Autodesk Inventor part; units mm, degrees
ref_plane "YZ Plane" through (0, 0, 0) normal (1, 0, 0) x (0, 1, 0)
ref_plane "XZ Plane" through (0, 0, 0) normal (0, 1, 0) x (-1, 0, 0)
ref_plane "XY Plane" through (0, 0, 0) normal (0, 0, 1) x (1, 0, 0)
sketch "Sketch1" plane through (0, 0, 0) normal (0, 0, 1) x (1, 0, 0)
  line L0 (0, 0) -> (30, 0)
  line L1 (0, 0) -> (0, 5)
  line L2 (0, 5) -> (30, 5)
  line L3 (30, 5) -> (30, 0)
  line L4 (30, 5) -> (30, 40)
  line L5 (30, 40) -> (33, 40)
  line L6 (33, 40) -> (33, 0)
  line L7 (33, 0) -> (30, 0)
  point P0 (23.0555, 5)
  dimension "d0" = 30
  dimension "d2" = 5
  dimension "d11" = 35
  dimension "d12" = 3
extrude "Extrusion1" add sketch "Sketch1" along normal blind 12
sketch "Sketch2" plane through (0, 0, 0) normal (0, -1, 0) x (1, 0, 0)
  circle A0 centre (25.8, 7) radius 2.125
  line L0 (33, 0) -> (33, 12)
  line L1 (0, 12) -> (33, 12)
  circle A1 centre (13.1, 7) radius 2.125
  point P0 (0, 0)
  point P1 (33, 6)
  dimension "d13" = 4.25
  dimension "d14" = 7.2
  dimension "d15" = 5
  dimension "d23" = 4.25
  dimension "d24" = 19.9
  dimension "d25" = 5
hole "Hole1" at (25.8, 0, 7) at (13.1, 0, 7) direction (0, 1, 0) diameter 5 end through all
properties part number "Support"
The model under review builds one solid part; all positions refer to its coordinate system, in mm. A direction names the side the tool comes from. Give positions to 0.01 mm unless a question says otherwise; leave off trailing zeros. Order: outer loops, then holes, each group sorted by start corner. A loop starts at its lowest first (then second) coordinate and runs counter-clockwise, first axis right, second up. Notation, with made-up numbers: (-39, 40) -> (-26, 40) arc R18 ccw to (-26, 56) -> close; hole circle Ø3 at (74, 24.25). An arc over 180 degrees is marked (long way). Write item = value, one per line. Start each with the question number.
(1) For L1, parallel to X at y = 2.85, z = 7; L2, parallel to Z at x = 13.1, y = 3.8; L3, parallel to X at y = 3.5, z = 5.25, list the stretches that pass through material, from the lowest coordinate up. Write a range as from..to.
(2) Take a section at D-D (y = 16). Write out the cut boundary in (x, z), plus the area to 3 significant figures.
(3) Take a section at B-B (z = 7). Write out the cut boundary in (x, y).
(4) Take a section at C-C (z = 1.25). Write out the cut boundary in (x, y).
(5) For pin 1 Ø3 at (x, z) = (13.1, 7) entering from -Y; pin 2 Ø6 at (y, z) = (31, 5.5) entering from -X; pin 3 Ø3.5 at (x, z) = (14, 8.5) entering from +Y, all flat-tipped, find the tip position at first contact; note any pin that passes through.
(6) Tool access review of faces 4 (the flat face through (30, 22, 6)), 5 (the flat face through (0, 2, 6)): name each direction out of +Z, -Z, +X, -X, +Y, -Y from which nothing blocks a thin tool from reaching the whole face with its end or side.
(7) Take a section at A-A (x = 25.8). Write out the cut boundary in (y, z).
(8) Draft analysis for pull direction Z (two halves, no side actions). For faces 1 (the cylindrical face through (12.349, 2.535, 4.615)), 2 (the flat face through (33, 20, 6)), 3 (the flat face through (23, 4, 0)), state which applies: +Z half, -Z half, draft (parallel to the pull), parting line (faces both ways), or undercut.
Returned:
q1.L1 = 0..10.6, 15.6..23.3, 28.3..33
q1.L2 = 0..4.5, 9.5..12
q1.L3 = 0..11.31, 14.89..24.01, 27.59..33
q2.outline = (30, 0) -> (33, 0) -> (33, 12) -> (30, 12) -> close
q2.area = 36.0 mm²
q3.outline = (0, 0) -> (10.6, 0) -> (10.6, 5) -> (0, 5) -> close; (15.6, 0) -> (23.3, 0) -> (23.3, 5) -> (15.6, 5) -> close; (28.3, 0) -> (33, 0) -> (33, 40) -> (30, 40) -> (30, 5) -> (28.3, 5) -> close
q4.outline = (0, 0) -> (33, 0) -> (33, 40) -> (30, 40) -> (30, 5) -> (0, 5) -> close
q5.pin_1 = through
q5.pin_2 = 30
q5.pin_3 = 5
q6.face_4 = +Z, -Z, -X, +Y
q6.face_5 = +Z, -Z, -X, +Y, -Y
q7.outline = (0, 0) -> (5, 0) -> (5, 4.5) -> (0, 4.5) -> close; (0, 9.5) -> (5, 9.5) -> (5, 12) -> (0, 12) -> close
q8.face_1 = undercut
q8.face_2 = draft
q8.face_3 = -Z half
